Input: part model. Units: mm. Frame: model coordinates. Face numbers are marked on the shaded views. A direction names the side the tool comes from. Round coordinates to 2 decimals unless told otherwise and drop trailing zeros. Loops run counter-clockwise (first coordinate to the right, second up) from the corner with the lowest first, then second, coordinate; pieces in that order, holes last. Notation, with made-up numbers: (-5.75, 26.5) - (17.25, 26.5) arc R16 cw to (17.25, 41.5) - close; hole circle Ø8 at (63.5, -4). An arc over 180 degrees is marked (long way). One line per question, with ' | ' between items. Start each with the question number.
Item 1: Section A-A, the plane x = 0. Return loops of the section in (y, z) (3 decimals).
Item 2: First-contact query: pin 1 (1 mm diameter, centred on x = 0, z = 1.5, fed in from -Y); pin 2 (2 mm diameter, centred on x = -8.5, y = 14.5, fed in from -Z); pin 3 (3.5 mm diameter, centred on x = 16.5, y = -12.5, fed in from -Z); pin 4 (8 mm diameter, centred on x = 1.5, y = 0, fed in from -Z). Flat tips, straight axial feed; report the tip coordinate or a pass-through.
Item 3: Set-up query: the marked faces 4 and 5. Return all of +Z, -Z, +X, -X, +Y, -Y with unobstructed straight access to the full face (end or side cutting, diameter ignored); none if empty.
Item 4: Draft query along Y for the marked faces 1, 2 and 3. Return one class per face: pulls with the +Y half, pulls with the -Y half, needs draft (parallel to the pull), parting line crosses it, or undercut.
Item 5: Material intervals for line 1 along Y through (x, z) = (0, 1.2) (3 decimals); line 2 along Y through (x, z) = (-18.5, 0.45); line 3 along Y through (x, z) = (7, 0.95), sorted ascending.
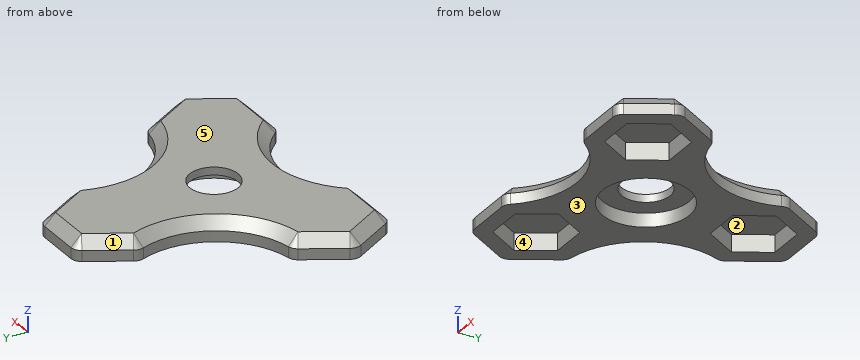
```python
from build123d import *

# Parameters (mm, degrees)
F1_DEPTH = 4
F2_R     = 8.075
F3_DEPTH = 2.55
F5_DEPTH = 3.2
F6_SIZE  = 1.99999
F7_R     = 4.5
F8_DEPTH = 25


# Not quite as in the source:
# - a fillet or chamfer is up to 0.001 mm smaller than in the source, because OpenCascade refuses the exact size


with BuildPart() as f1:
    # F0 (on Top) → F1 (new body)
    with BuildSketch(Plane.XY):
        with BuildLine():
            Line((-5.7735026919, 28), (-9.9042445516, 20.8453452261))
            ThreePointArc((-9.9042445516, 20.8453452261), (-10.1650850266, 20.0138217399), (-10.0475406836, 19.1503100787))
            ThreePointArc((-10.0475406836, 19.1503100787), (-11.1235598668, 6.4221902835), (-21.6084253603, -0.8737295618))
            ThreePointArc((-21.6084253603, -0.8737295618), (-22.4150205669, -1.2036890053), (-23.0047207922, -1.8453452261))
            Line((-23.0047207922, -1.8453452261), (-27.1354626519, -9))
            ThreePointArc((-27.1354626519, -9), (-27.4034118443, -10), (-27.1354626519, -11))
            Line((-27.1354626519, -11), (-23.0940107676, -18))
            ThreePointArc((-23.0940107676, -18), (-22.36195996, -18.7320508076), (-21.36195996, -19))
            Line((-21.36195996, -19), (-13.1004762407, -19))
            ThreePointArc((-13.1004762407, -19), (-12.2499355402, -18.8101327346), (-11.5608846767, -18.2765805169))
            ThreePointArc((-11.5608846767, -18.2765805169), (0, -12.8443805669), (11.5608846767, -18.2765805169))
            ThreePointArc((11.5608846767, -18.2765805169), (12.2499355402, -18.8101327346), (13.1004762407, -19))
            Line((13.1004762407, -19), (21.36195996, -19))
            ThreePointArc((21.36195996, -19), (22.36195996, -18.7320508076), (23.0940107676, -18))
            Line((23.0940107676, -18), (27.1354626519, -11))
            ThreePointArc((27.1354626519, -11), (27.4034118443, -10), (27.1354626519, -9))
            Line((27.1354626519, -9), (23.0047207922, -1.8453452261))
            ThreePointArc((23.0047207922, -1.8453452261), (22.4150205669, -1.2036890053), (21.6084253603, -0.8737295618))
            ThreePointArc((21.6084253603, -0.8737295618), (11.1235598668, 6.4221902835), (10.0475406836, 19.1503100787))
            ThreePointArc((10.0475406836, 19.1503100787), (10.1650850266, 20.0138217399), (9.9042445516, 20.8453452261))
            Line((9.9042445516, 20.8453452261), (5.7735026919, 28))
            ThreePointArc((5.7735026919, 28), (5.0414518843, 28.7320508076), (4.0414518843, 29))
            Line((4.0414518843, 29), (-4.0414518843, 29))
            ThreePointArc((-4.0414518843, 29), (-5.0414518843, 28.7320508076), (-5.7735026919, 28))
        make_face()
    extrude(amount=F1_DEPTH)

    # F2 (on face) → F3 (cut)
    with BuildSketch(Plane.XY):
        Circle(F2_R)
    extrude(amount=F3_DEPTH, mode=Mode.SUBTRACT)

    # F4 (on face) → F5 (cut)
    with BuildSketch(Plane.XY):
        Polygon((6.9282032303, 20), (3.4641016151, 26), (-3.4641016151, 26), (-6.9282032303, 20), (-3.4641016151, 14), (3.4641016151, 14), align=None)
        Polygon((-13.8564064606, -16), (-10.3923048454, -10), (-13.8564064606, -4), (-20.7846096908, -4), (-24.248711306, -10), (-20.7846096908, -16), align=None)
        Polygon((20.7846096908, -4), (13.8564064606, -4), (10.3923048454, -10), (13.8564064606, -16), (20.7846096908, -16), (24.248711306, -10), align=None)
    extrude(amount=F5_DEPTH, mode=Mode.SUBTRACT)

    # F6 (size 2 in the source; OpenCascade refuses exactly that, so slightly less here)
    f6_edges = [f1.edges().sort_by_distance(p)[0] for p in [
        (10.165085, 20.013822, 4),
        (7.838874, 24.422673, 4),
        (5.041452, 28.732051, 4),
        (0, 29, 4),
        (-5.041452, 28.732051, 4),
        (-7.838874, 24.422673, 4),
        (-10.165085, 20.013822, 4),
        (-11.12356, 6.42219, 4),
        (-22.415021, -1.203689, 4),
        (-25.070092, -5.422673, 4),
        (-27.403412, -10, 4),
        (-25.114737, -14.5, 4),
        (-22.36196, -18.732051, 4),
        (-17.231218, -19, 4),
        (-12.249936, -18.810133, 4),
        (0, -12.844381, 4),
        (12.249936, -18.810133, 4),
        (17.231218, -19, 4),
        (22.36196, -18.732051, 4),
        (25.114737, -14.5, 4),
        (27.403412, -10, 4),
        (25.070092, -5.422673, 4),
        (22.415021, -1.203689, 4),
        (11.12356, 6.42219, 4),
    ]]
    chamfer(f6_edges, length=F6_SIZE)

    # F7 (on face) → F8 (cut)
    with BuildSketch(Plane.XY.offset(4)):
        Circle(F7_R)
    extrude(amount=-F8_DEPTH, mode=Mode.SUBTRACT)


solid = f1.part
```
Return value:
1) outline: (-12.844, 0) - (-8.075, 0) - (-8.075, 2.55) - (-4.5, 2.55) - (-4.5, 4) - (-10.844, 4) - (-12.844, 2) - close; (4.5, 2.55) - (8.075, 2.55) - (8.075, 0) - (14, 0) - (14, 3.2) - (26, 3.2) - (26, 0) - (29, 0) - (29, 2) - (27, 4) - (4.5, 4) - close
2) pin 1: y = -12.85 | pin 2: z = 0 | pin 3: z = 3.2 | pin 4: z = 2.55
3) face 4: -Z | face 5: +Z, +X, -X, +Y, -Y
4) face 1: pulls with the +Y half | face 2: undercut | face 3: needs draft
5) line 1: -12.844 to -8.075, 8.075 to 14, 26 to 29 | line 2: -19 to -16, -4 to 0.01 | line 3: -14.58 to -4.03, 4.03 to 25.88
